Source: CAD feature listing. Evaluate the final solid. Frame: model axes, mm. A direction names the side the tool comes from. Give positions to 0.01 mm unless a question says otherwise; leave off trailing zeros. Loops run counter-clockwise (first coordinate to the right, second up) from the corner with the lowest first, then second, coordinate; pieces in that order, holes last. Notation, with made-up numbers: (74.5, 88.25) - (90.5, 88.25) arc R11 ccw to (90.5, 109.25) - close; hole circle Ø7 at (-21, 67.25). An arc over 180 degrees is marked (long way). Write each question's results on one line, items separated by ' | '. Start each with the question number.
(1) Cut plane D-D on y = 3.8. Return the cut outline in (x, z), then the cut area to 3 significant figures.
(2) Contact query for flat-ended pins moving along their axis: pin 1 (5.5 mm diameter, centred on x = 0, z = 0, fed in from +Y); pin 2 (1.5 mm diameter, centred on y = 5, z = 2, fed in from +X); pin 3 (2.5 mm diameter, centred on x = 7.5, z = 0, fed in from +Y). Output: stop coordinate, or through.
(3) Cut plane B-B on x = 0. Return the cut outline in (y, z), then the cut area to 4 significant figures.
(4) Reachability of faces 1 (the cylindrical face through (0.9, 2.71, 2.86)), 2 (the cylindrical face through (4.214, 3.726, -0.553)) from +Z, -Z, +X, -X, +Y, -Y: full face, straight path, thin tool, end or side. Return the list, or none.
(5) Pull-direction query (X, two-part tool) for faces 3 (the flat face through (0, 2, 5)), 4 (the cylindrical face through (3.2, 1, 10)), 5 (the cylindrical face through (0.03, 1.01, -8.25)); classes: pulls with the +X half, pulls with the -X half, needs draft (parallel to the pull), parting line crosses it, or undercut.
(6) Cut plane C-C on z = -7.5. Return the cut outline in (x, y), then the cut area to 3 significant figures.
(7) Material intervals for line 1 along X through (y, z) = (0.9, 0); line 2 along X through (y, z) = (2.8, 0); line 3 along Y through (x, z) = (-6.5, -0.75), sorted ascending. Write a range as [from, to].
(8) Cut plane A-A on z = 0. Return the cut outline in (x, y).
from build123d import *

# Parameters (mm, degrees)
SKIZZE1_R                       = 10.5
AUFSATZ_LINEAR_AUSTRAGEN1_DEPTH = 2
SKIZZE2_R                       = 4.25
SKIZZE2_R_2                     = 3
AUFSATZ_LINEAR_AUSTRAGEN2_DEPTH = 3.5
SKIZZE3_R                       = 0.75
SCHNITT_LINEAR_AUSTRAGEN1_DEPTH = 3.5
SCHNITT_LINEAR_START            = -3.5
SKIZZE4_R                       = 3
SCHNITT_LINEAR_AUSTRAGEN2_DEPTH = 3.5


with BuildPart() as part:
    # Skizze1 → Aufsatz-Linear austragen1 (new body)
    with BuildSketch(Plane(origin=(0, 0, 0), x_dir=(1, 0, 0), z_dir=(0, 1, 0))):
        with Locations(Location((0, 0, 0), (0, 0, 270))):
            Circle(SKIZZE1_R)
    extrude(amount=AUFSATZ_LINEAR_AUSTRAGEN1_DEPTH)

    # Skizze2 → Aufsatz-Linear austragen2 (add)
    with BuildSketch(Plane(origin=(0, 2, 0), x_dir=(1, 0, 0), z_dir=(0, 1, 0))):
        with Locations(Location((0, 0, 0), (0, 0, 270))):
            Circle(SKIZZE2_R)
        with Locations(Location((0, 0, 0), (0, 0, 270))):
            Circle(SKIZZE2_R_2, mode=Mode.SUBTRACT)
    extrude(amount=AUFSATZ_LINEAR_AUSTRAGEN2_DEPTH)

    # Skizze3 → Schnitt-Linear austragen1 (cut)
    with BuildSketch(Plane(origin=(0, 2, 0), x_dir=(1, 0, 0), z_dir=(0, 1, 0))):
        with Locations(Location((0, 7.5, 0), (0, 0, 270))):
            Circle(SKIZZE3_R)
        with Locations(Location((0, -7.5, 0), (0, 0, 270))):
            Circle(SKIZZE3_R)
        with Locations(Location((7.5, 0, 0), (0, 0, 270))):
            Circle(SKIZZE3_R)
        with Locations(Location((-7.5, 0, 0), (0, 0, 270))):
            Circle(SKIZZE3_R)
    extrude(amount=-SCHNITT_LINEAR_AUSTRAGEN1_DEPTH, mode=Mode.SUBTRACT)

    # Skizze4 → Schnitt-Linear austragen2 (cut)
    with BuildSketch(Plane(origin=(0, 2, 0), x_dir=(1, 0, 0), z_dir=(0, 1, 0)).offset(SCHNITT_LINEAR_START)):
        with Locations(Location((0, 0, 0), (0, 0, 270))):
            Circle(SKIZZE4_R)
    extrude(amount=SCHNITT_LINEAR_AUSTRAGEN2_DEPTH, mode=Mode.SUBTRACT)


solid = part.part
Ans:
1) outline: circle Ø8.5 at (0, 0); hole circle Ø6 at (0, 0) | area: 28.5 mm^2
2) pin 1: through | pin 2: x = 4.06 | pin 3: y = 2
3) outline: (0, -10.5) - (2, -10.5) - (2, -8.25) - (0, -8.25) - close; (0, -6.75) - (2, -6.75) - (2, -4.25) - (5.5, -4.25) - (5.5, -3) - (0, -3) - close; (0, 3) - (5.5, 3) - (5.5, 4.25) - (2, 4.25) - (2, 6.75) - (0, 6.75) - close; (0, 8.25) - (2, 8.25) - (2, 10.5) - (0, 10.5) - close | area: 32.75 mm^2
4) face 1: +Y, -Y | face 2: +Y
5) face 3: needs draft | face 4: parting line crosses it | face 5: undercut
6) outline: (-7.35, 0) - (-0.75, 0) - (-0.75, 2) - (-7.35, 2) - close; (0.75, 0) - (7.35, 0) - (7.35, 2) - (0.75, 2) - close | area: 26.4 mm^2
7) line 1: [-10.5, -8.25], [-6.75, -3], [3, 6.75], [8.25, 10.5] | line 2: [-4.25, -3], [3, 4.25] | line 3: [0, 2]
8) outline: (-10.5, 0) - (-8.25, 0) - (-8.25, 2) - (-10.5, 2) - close; (-6.75, 0) - (-3, 0) - (-3, 5.5) - (-4.25, 5.5) - (-4.25, 2) - (-6.75, 2) - close; (3, 0) - (6.75, 0) - (6.75, 2) - (4.25, 2) - (4.25, 5.5) - (3, 5.5) - close; (8.25, 0) - (10.5, 0) - (10.5, 2) - (8.25, 2) - close
